```python
from build123d import *

# Parameters (mm, degrees)
F0_W     = 84
F0_H     = 64
F1_DEPTH = 1
F2_R     = 4.25
F3_DEPTH = 1
F4_R     = 1.75
F5_DEPTH = 40


with BuildPart() as f1:
    # F0 (on Top) → F1 (new body)
    with BuildSketch(Plane.XY):
        Rectangle(F0_W, F0_H)
    extrude(amount=F1_DEPTH)

    # F2 (on face) → F3 (join)
    with BuildSketch(Plane(origin=(0, 0, 0), x_dir=(1, 0, 0), z_dir=(0, 0, -1))):
        with Locations((-39, 29)):
            Circle(F2_R)
        with Locations((-39, -29)):
            Circle(F2_R)
        with Locations((39, -29)):
            Circle(F2_R)
        with Locations((39, 29)):
            Circle(F2_R)
    extrude(amount=-F3_DEPTH)

    # F4 (on face) → F5 (cut)
    with BuildSketch(Plane.XY.offset(1)):
        with Locations((-39, 29)):
            Circle(F4_R)
        with Locations((39, 29)):
            Circle(F4_R)
        with Locations((-39, -29)):
            Circle(F4_R)
        with Locations((39, -29)):
            Circle(F4_R)
    extrude(amount=-F5_DEPTH, mode=Mode.SUBTRACT)


solid = f1.part
```
Geometry check sheet. Reference: the model listing, model coordinates, mm. Coordinates: 2 decimals unless noted, no trailing zeros. Write each loop counter-clockwise with the first axis right and the second up, starting at its lowest first coordinate (ties: lowest second). Pieces come first, ordered by that corner, then holes. Notation, with made-up numbers: M 75.5,8 L 115.5,8 A29 cw 115.5,41 Z; hole C 84.25,83.5 d7. An arc over 180 degrees is marked long. Use one line per item in the form item = value. Start each with the question number.
1) Section check C-C on z = 0.6. Enter the section's corners in (x, y), and give its area (3 significant figures).
2) Section check A-A on x = -39. Enter the section's corners in (y, z), and give its area (3 significant figures).
3) Section check D-D on y = -21. Enter the section's corners in (x, z), and give its area (3 significant figures).
4) Go/stop test with flat-tipped pins: pin 1 Ø0.5 at (y, z) = (-1, 0.5) entering from +X; pin 2 Ø4 at (x, y) = (-39, 29) entering from -Z; pin 3 Ø3 at (x, y) = (-39, -29) entering from -Z. Record where each tip stops, or that it passes through.
5) Release check for a two-part mould opening along Y. For faces 1 (the cylindrical face through (41.94, 32.07, 0.49)), 2 (the flat face through (-1, 0, 0)) record: pulls with the +Y half, pulls with the -Y half, needs draft (parallel to the pull), parting line crosses it, or undercut.
6) Section check B-B on y = 29. Enter the section's corners in (x, z), and give its area (3 significant figures).
7) Thickness scan on probe 1 along Y at (x, z) = (39, 0.7); probe 2 along Y at (x, z) = (26, 0.25); probe 3 along X at (y, z) = (-18, 0.9). Record the ranges inside material, lowest first. Write a range as from..to.
Responses:
q1.outline = M -42,-25.99 A4.25 ccw -35.99,-32 L 35.99,-32 A4.25 ccw 42,-25.99 L 42,25.99 A4.25 ccw 35.99,32 L -35.99,32 A4.25 ccw -42,25.99 Z; hole C -39,-29 d3.5; hole C -39,29 d3.5; hole C 39,-29 d3.5; hole C 39,29 d3.5
q1.area = 5,380 mm2
q2.outline = M -33.25,0 L -30.75,0 L -30.75,1 L -33.25,1 Z; M -27.25,0 L 27.25,0 L 27.25,1 L -27.25,1 Z; M 30.75,0 L 33.25,0 L 33.25,1 L 30.75,1 Z
q2.area = 59.5 mm2
q3.outline = M -42,0 L 42,0 L 42,1 L -42,1 Z
q3.area = 84.0 mm2
q4.pin_1 = 42
q4.pin_2 = 0
q4.pin_3 = through
q5.face_1 = undercut
q5.face_2 = needs draft
q6.outline = M -43.25,0 L -40.75,0 L -40.75,1 L -43.25,1 Z; M -37.25,0 L 37.25,0 L 37.25,1 L -37.25,1 Z; M 40.75,0 L 43.25,0 L 43.25,1 L 40.75,1 Z
q6.area = 79.5 mm2
q7.probe_1 = -33.25..-30.75, -27.25..27.25, 30.75..33.25
q7.probe_2 = -32..32
q7.probe_3 = -42..42
